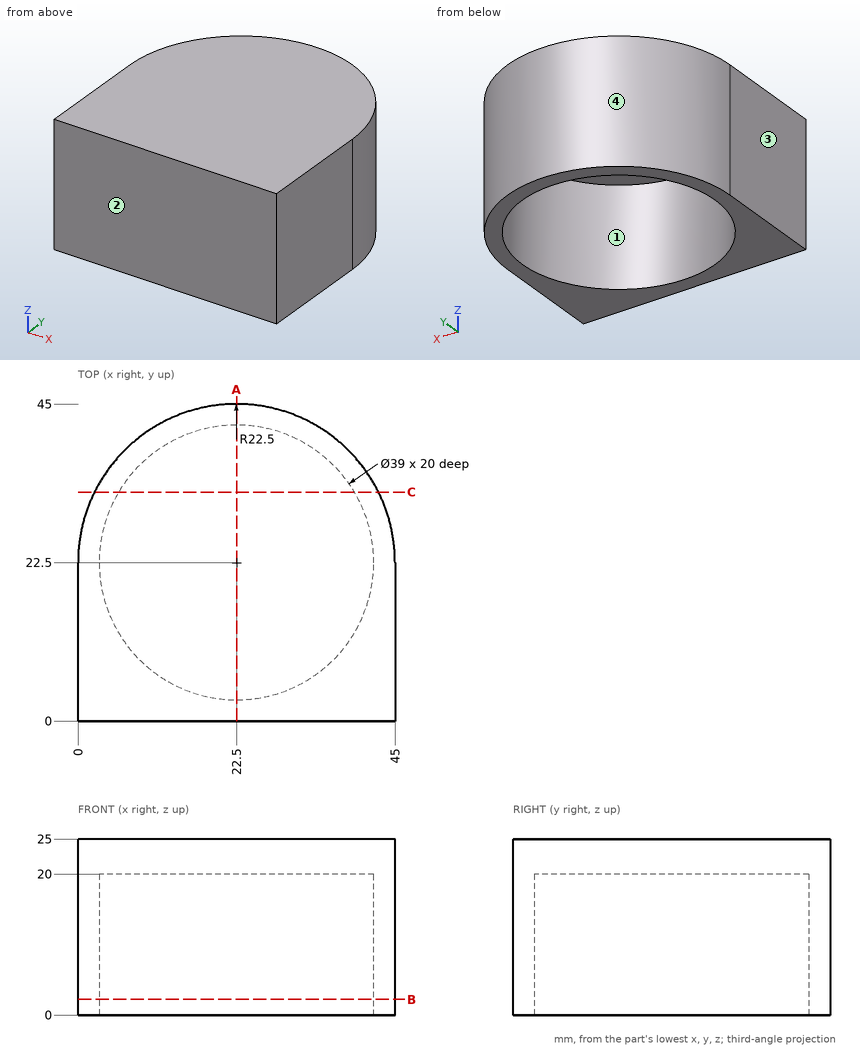
Answer from the drawing. Dimensions are ordinates in mm from the lowest x, y and z of the part. Coordinates: 2 decimals unless noted, no trailing zeros. Order: outer loops, then holes, each group sorted by start corner. A loop starts at its lowest first (then second) coordinate and runs counter-clockwise, first axis right, second up. Notation, with made-up numbers: (64, 70) -> (119, 70) arc R25 ccw to (119, 82) -> close; hole circle Ø7 at (25.25, 3.5). An arc over 180 degrees is marked (long way). Answer as a JSON object with one key per item and string values.
1) A cutting plane is placed at A-A, the plane x = 22.5. Determine the outline of the cut face in (y, z).
Model answer:
{"outline": "(0, 0) -> (3, 0) -> (3, 20) -> (42, 20) -> (42, 0) -> (45, 0) -> (45, 25) -> (0, 25) -> close"}
2) A cutting plane is placed at B-B, the plane z = 2.25. Determine the outline of the cut face in (x, y).
Model answer:
{"outline": "(0, 0) -> (45, 0) -> (45, 22.5) arc R22.5 ccw to (0, 22.5) -> close; hole circle Ø39 at (22.5, 22.5)"}
3) The mould has two halves that part along X. Classify the marked faces 1, 2, 3 and 4: released by +X, released by -X, zero draft, split by the parting line, or undercut.
Model answer:
{"face 1": "undercut", "face 2": "zero draft", "face 3": "released by -X", "face 4": "split by the parting line"}
4) Each of these flat-tipped pins is pushed along its axis until it touches: pin 1 (1 mm diameter, centred on y = 24.5, z = 21, fed in from -X); pin 2 (12 mm diameter, centred on x = 27.5, z = 18, fed in from +Y); pin 3 (1.5 mm diameter, centred on x = 24.5, y = 8, fed in from -Z). Where does it stop, or does it pass through?
Model answer:
{"pin 1": "stops at x = 0.05", "pin 2": "stops at y = 45", "pin 3": "stops at z = 20"}
5) Consider line 1 along Y through (x, z) = (23, 13.25); line 2 along Z through (x, y) = (18, 9); line 3 along Y through (x, z) = (17, 13.5). Determine where each line is inside the solid, lowest interval first. Write a range as from..to.
Model answer:
{"line 1": "y = 0..3.01, 41.99..44.99", "line 2": "z = 20..25", "line 3": "y = 0..3.79, 41.21..44.32"}
6) A cutting plane is placed at C-C, the plane y = 32.5. Determine the outline of the cut face in (x, z), plus the area to 3 significant figures.
Model answer:
{"outline": "(2.34, 0) -> (5.76, 0) -> (5.76, 20) -> (39.24, 20) -> (39.24, 0) -> (42.66, 0) -> (42.66, 25) -> (2.34, 25) -> close", "area": "338 mm²"}
